For this review, take the finished solid that the model builds, in its own axes (mm). Face numbers are marked on the shaded views. A direction names the side the tool comes from. Coordinates: 2 decimals unless noted, no trailing zeros. Loops run counter-clockwise (first coordinate to the right, second up) from the corner with the lowest first, then second, coordinate; pieces in that order, holes last. Notation, with made-up numbers: (29.25, 9) -> (37.25, 9) arc R18 cw to (37.25, 20) -> close; hole circle Ø11 at (46, 8). An arc over 180 degrees is marked (long way). Answer in a Markdown table with one row per item.
from build123d import *

# Parameters (mm, degrees)
BOSS_EXTRUDE1_DEPTH = 12
SHELL1_T            = -1
SKETCH3_R           = 3
SKETCH3_R_2         = 2
CUT_EXTRUDE1_DEPTH  = 12
SKETCH4_W           = 10
SKETCH4_H           = 10
CUT_EXTRUDE2_DEPTH  = 12
FILLET1_R           = 2


with BuildPart() as part:
    # Sketch2 → Boss-Extrude1 (new body)
    with BuildSketch(Plane.XY):
        Polygon((-28.002919882, 3.210239845), (-126.301165196, -65.618932518), (-126.301165196, -94.618932518), (-114.301165196, -94.618932518), (-114.301165196, -71.722772739), (-24.421364281, -8.788258605), (18.577059182, -8.788258605), (119.718098707, -67.182065001), (125.718098707, -56.789760155), (21.795050253, 3.210239845), align=None)
    extrude(amount=BOSS_EXTRUDE1_DEPTH)

    # Shell1
    shell1_openings = [part.faces().sort_by_distance(p)[0] for p in [
        (-120.301165196, -94.618932518, 6),
    ]]
    offset(amount=SHELL1_T, openings=shell1_openings, kind=Kind.INTERSECTION)

    # Sketch3 → Cut-Extrude1 (cut)
    with BuildSketch(Plane.XY.offset(12)):
        with Locations((-2.922152549, -2.788258605)):
            Circle(SKETCH3_R)
        with Locations((117.521946284, -58.985912578)):
            Circle(SKETCH3_R_2)
    extrude(amount=-CUT_EXTRUDE1_DEPTH, mode=Mode.SUBTRACT)

    # Sketch4 → Cut-Extrude2 (cut)
    with BuildSketch(Plane(origin=(118.879261515, -68.634973637, 0), x_dir=(0, 0, -1), z_dir=(0.8660254037844357, -0.500000000000005, 0))):
        with Locations((-6.037142442, 7.633616623)):
            Rectangle(SKETCH4_W, SKETCH4_H)
    extrude(amount=-CUT_EXTRUDE2_DEPTH, mode=Mode.SUBTRACT)

    # Fillet1
    # the kernel refuses this fillet: 2 mm, written as the material it takes off along each edge
    with BuildSketch(Plane(origin=(119.718098707, -67.182065001, -5), x_dir=(0.499999999999999, 0.8660254037844393, 0), z_dir=(0, 0, 1)), Plane(origin=(125.718098707, -56.789760155, -5), x_dir=(-0.8660254037844393, 0.499999999999999, 0), z_dir=(0, 0, 1))) as fillet1_piece_1:
        with BuildLine():
            CenterArc((FILLET1_R, FILLET1_R), FILLET1_R, 180, 90)
            Line((0, FILLET1_R), (0, 0))
            Line((0, 0), (FILLET1_R, 0))
        make_face()
    extrude(amount=22, mode=Mode.SUBTRACT)


solid = part.part
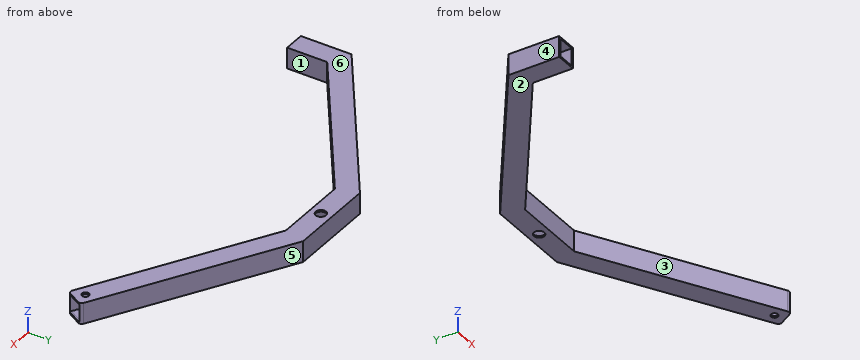
Item 1: For the marked faces 1 and 2, list the 3-axis set-ups (+Z, -Z, +X, -X, +Y, -Y) from which the entire face can be reached by the end or side of a thin tool; tool diameter is ignored.
Worked answers:
| item | result |
|---|---|
| face 1 | +Z, -Z, +X, -Y |
| face 2 | -Z, +X, -X, +Y, -Y |
Item 2: Insertion check: pin 1 (2 mm diameter, centred on x = -1.5, z = 5, fed in from -Y); pin 2 (4 mm diameter, centred on y = -33.5, z = 8.5, fed in from -X); pin 3 (5 mm diameter, centred on y = -81.5, z = 6.5, fed in from +X). Each pin has a flat end and moves straight along its axis. Give the tip position at first contact, or say it passes through.
Worked answers:
| item | result |
|---|---|
| pin 1 | y = -8.79 |
| pin 2 | x = -83.29 |
| pin 3 | x = -114.3 |
Item 3: Take a section at B-B, the plane y = -41. State the section outline as (x, z) points.
Worked answers:
| item | result |
|---|---|
| outline | (-91.14, 0) -> (-70.42, 0) -> (-70.42, 12) -> (-91.14, 12) -> close; (74.37, 0) -> (98.37, 0) -> (98.37, 12) -> (74.37, 12) -> close; hole (-89.4, 1) -> (-72.17, 1) -> (-72.17, 11) -> (-89.4, 11) -> close; hole (76.37, 1) -> (96.37, 1) -> (96.37, 11) -> (76.37, 11) -> close |
Item 4: Take a section at A-A, the plane x = -11.5. State the section outline as (y, z) points, and give its area (3 significant figures).
Worked answers:
| item | result |
|---|---|
| outline | (-8.79, 0) -> (3.21, 0) -> (3.21, 12) -> (-8.79, 12) -> close; hole (-7.79, 1) -> (2.21, 1) -> (2.21, 11) -> (-7.79, 11) -> close |
| area | 44.0 mm² |
Item 5: The part is to be moulded in two halves that separate along X. For the marked faces 3, 4, 5 and 6, say which applies: +X half, -X half, draft (parallel to the pull), parting line (faces both ways), or undercut.
Worked answers:
| item | result |
|---|---|
| face 3 | undercut |
| face 4 | -X half |
| face 5 | +X half |
| face 6 | draft |
Item 6: For L1, parallel to X at y = -46.5, z = 3.5; L2, parallel to Z at x = -116, y = -90; L3, parallel to X at y = -56.5, z = 8, list the stretches that pass through material, from the lowest coordinate up.
Worked answers:
| item | result |
|---|---|
| L1 | -99 to -97.25, -80.02 to -78.28, 83.9 to 85.9, 105.9 to 107.9 |
| L2 | 0 to 1, 11 to 12 |
| L3 | -113.28 to -111.53, -94.3 to -92.56, 101.22 to 103.22, 123.22 to 124.71 |
Item 7: Take a section at C-C, the plane y = -74. State the section outline as (x, z) points.
Worked answers:
| item | result |
|---|---|
| outline | (-126.3, 0) -> (-114.3, 0) -> (-114.3, 12) -> (-126.3, 12) -> close; hole (-125.3, 1) -> (-115.3, 1) -> (-115.3, 11) -> (-125.3, 11) -> close |
